CAD build for the part. Positions are in the model's coordinates, mm. A direction names the side the tool comes from. Coordinates: 2 decimals unless noted, no trailing zeros. Loops run counter-clockwise (first coordinate to the right, second up) from the corner with the lowest first, then second, coordinate; pieces in that order, holes last. Notation, with made-up numbers: (-33, 6.5) -> (-16, 6.5) arc R28 cw to (-16, 39.5) -> close; hole circle Ø5 at (78.25, 62.25). An arc over 180 degrees is marked (long way). Write each question's results on one line, items separated by ' | '.
from build123d import *

# Parameters (mm, degrees)
F0_W     = 74.25791291
F0_H     = 4.7
F0_W_2   = 3.271043545
F0_W_3   = 1.428956455
F0_H_2   = 8.3906837511
F0_H_3   = 13.5
F0_H_4   = 7.9193162489
F1_DEPTH = 27.2
F2_W     = 39.9343147874
F2_H     = 22.3026155613
F3_DEPTH = 155


with BuildPart() as f1:
    # F0 (on Top) → F1 (new body)
    with BuildSketch(Plane.XY):
        Polygon((-41.828956455, 87.5000014901), (-41.828956455, 74.9143162489), (-40.4, 74.9143162489), (-40.4, 83.305), (-37.128956455, 83.305), (-37.128956455, 87.5000014901), align=None)
        with Locations((0, 72.5643162489)):
            Rectangle(F0_W, F0_H)
        with Locations((-38.7644782275, 72.5643162489)):
            Rectangle(F0_W_2, F0_H)
        with Locations((-41.1144782275, 72.5643162489)):
            Rectangle(F0_W_3, F0_H)
        with Locations((38.7644782275, 79.1096581244)):
            Rectangle(F0_W_2, F0_H_2)
        Polygon((37.128956455, 87.5000014901), (37.128956455, 83.305), (40.4, 83.305), (40.4, 74.9143162489), (41.828956455, 74.9143162489), (41.828956455, 87.5000014901), align=None)
        with Locations((38.7644782275, 72.5643162489)):
            Rectangle(F0_W_2, F0_H)
        with Locations((41.1144782275, 72.5643162489)):
            Rectangle(F0_W_3, F0_H)
        with Locations((-41.1144782275, 63.4643162489)):
            Rectangle(F0_W_3, F0_H_3)
        with Locations((-38.7644782275, 63.4643162489)):
            Rectangle(F0_W_2, F0_H_3)
        with Locations((38.7644782275, 63.4643162489)):
            Rectangle(F0_W_2, F0_H_3)
        with Locations((41.1144782275, 63.4643162489)):
            Rectangle(F0_W_3, F0_H_3)
        with Locations((41.1144782275, 54.3643162489)):
            Rectangle(F0_W_3, F0_H)
        with Locations((38.7644782275, 54.3643162489)):
            Rectangle(F0_W_2, F0_H)
        with Locations((0, 54.3643162489)):
            Rectangle(F0_W, F0_H)
        with Locations((-41.1144782275, 54.3643162489)):
            Rectangle(F0_W_3, F0_H)
        with Locations((-38.7644782275, 54.3643162489)):
            Rectangle(F0_W_2, F0_H)
        with Locations((-41.1144782275, 45.2643162489)):
            Rectangle(F0_W_3, F0_H_3)
        with Locations((-38.7644782275, 45.2643162489)):
            Rectangle(F0_W_2, F0_H_3)
        with Locations((38.7644782275, 45.2643162489)):
            Rectangle(F0_W_2, F0_H_3)
        with Locations((41.1144782275, 45.2643162489)):
            Rectangle(F0_W_3, F0_H_3)
        with Locations((-41.1144782275, 36.1643162489)):
            Rectangle(F0_W_3, F0_H)
        with Locations((-38.7644782275, 36.1643162489)):
            Rectangle(F0_W_2, F0_H)
        with Locations((0, 36.1643162489)):
            Rectangle(F0_W, F0_H)
        with Locations((38.7644782275, 36.1643162489)):
            Rectangle(F0_W_2, F0_H)
        with Locations((41.1144782275, 36.1643162489)):
            Rectangle(F0_W_3, F0_H)
        with Locations((-41.1144782275, 27.0643162489)):
            Rectangle(F0_W_3, F0_H_3)
        with Locations((-38.7644782275, 27.0643162489)):
            Rectangle(F0_W_2, F0_H_3)
        with Locations((38.7644782275, 27.0643162489)):
            Rectangle(F0_W_2, F0_H_3)
        with Locations((41.1144782275, 27.0643162489)):
            Rectangle(F0_W_3, F0_H_3)
        with Locations((-41.1144782275, 17.9643162489)):
            Rectangle(F0_W_3, F0_H)
        with Locations((-38.7644782275, 17.9643162489)):
            Rectangle(F0_W_2, F0_H)
        with Locations((0, 17.9643162489)):
            Rectangle(F0_W, F0_H)
        with Locations((38.7644782275, 17.9643162489)):
            Rectangle(F0_W_2, F0_H)
        with Locations((41.1144782275, 17.9643162489)):
            Rectangle(F0_W_3, F0_H)
        with Locations((-41.1144782275, 8.8643162489)):
            Rectangle(F0_W_3, F0_H_3)
        with Locations((-38.7644782275, 8.8643162489)):
            Rectangle(F0_W_2, F0_H_3)
        with Locations((-41.1144782275, -0.2356837511)):
            Rectangle(F0_W_3, F0_H)
        with Locations((-38.7644782275, -0.2356837511)):
            Rectangle(F0_W_2, F0_H)
        with Locations((0, -0.2356837511)):
            Rectangle(F0_W, F0_H)
        with Locations((38.7644782275, 8.8643162489)):
            Rectangle(F0_W_2, F0_H_3)
        with Locations((41.1144782275, 8.8643162489)):
            Rectangle(F0_W_3, F0_H_3)
        with Locations((38.7644782275, -0.2356837511)):
            Rectangle(F0_W_2, F0_H)
        with Locations((41.1144782275, -0.2356837511)):
            Rectangle(F0_W_3, F0_H)
        with Locations((-41.1144782275, -9.3356837511)):
            Rectangle(F0_W_3, F0_H_3)
        with Locations((-38.7644782275, -9.3356837511)):
            Rectangle(F0_W_2, F0_H_3)
        with Locations((-41.1144782275, -18.4356837511)):
            Rectangle(F0_W_3, F0_H)
        with Locations((-38.7644782275, -18.4356837511)):
            Rectangle(F0_W_2, F0_H)
        with Locations((0, -18.4356837511)):
            Rectangle(F0_W, F0_H)
        with Locations((38.7644782275, -9.3356837511)):
            Rectangle(F0_W_2, F0_H_3)
        with Locations((41.1144782275, -9.3356837511)):
            Rectangle(F0_W_3, F0_H_3)
        with Locations((38.7644782275, -18.4356837511)):
            Rectangle(F0_W_2, F0_H)
        with Locations((41.1144782275, -18.4356837511)):
            Rectangle(F0_W_3, F0_H)
        with Locations((-41.1144782275, -27.5356837511)):
            Rectangle(F0_W_3, F0_H_3)
        with Locations((-38.7644782275, -27.5356837511)):
            Rectangle(F0_W_2, F0_H_3)
        with Locations((38.7644782275, -27.5356837511)):
            Rectangle(F0_W_2, F0_H_3)
        with Locations((41.1144782275, -27.5356837511)):
            Rectangle(F0_W_3, F0_H_3)
        with Locations((-41.1144782275, -36.6356837511)):
            Rectangle(F0_W_3, F0_H)
        with Locations((-38.7644782275, -36.6356837511)):
            Rectangle(F0_W_2, F0_H)
        with Locations((0, -36.6356837511)):
            Rectangle(F0_W, F0_H)
        with Locations((38.7644782275, -36.6356837511)):
            Rectangle(F0_W_2, F0_H)
        with Locations((41.1144782275, -36.6356837511)):
            Rectangle(F0_W_3, F0_H)
        with Locations((-41.1144782275, -45.7356837511)):
            Rectangle(F0_W_3, F0_H_3)
        with Locations((-38.7644782275, -45.7356837511)):
            Rectangle(F0_W_2, F0_H_3)
        with Locations((-41.1144782275, -54.8356837511)):
            Rectangle(F0_W_3, F0_H)
        with Locations((-38.7644782275, -54.8356837511)):
            Rectangle(F0_W_2, F0_H)
        with Locations((0, -54.8356837511)):
            Rectangle(F0_W, F0_H)
        with Locations((38.7644782275, -54.8356837511)):
            Rectangle(F0_W_2, F0_H)
        with Locations((41.1144782275, -54.8356837511)):
            Rectangle(F0_W_3, F0_H)
        with Locations((38.7644782275, -45.7356837511)):
            Rectangle(F0_W_2, F0_H_3)
        with Locations((41.1144782275, -45.7356837511)):
            Rectangle(F0_W_3, F0_H_3)
        with Locations((-41.1144782275, -63.9356837511)):
            Rectangle(F0_W_3, F0_H_3)
        with Locations((-38.7644782275, -63.9356837511)):
            Rectangle(F0_W_2, F0_H_3)
        with Locations((38.7644782275, -63.9356837511)):
            Rectangle(F0_W_2, F0_H_3)
        with Locations((41.1144782275, -63.9356837511)):
            Rectangle(F0_W_3, F0_H_3)
        with Locations((-41.1144782275, -73.0356837511)):
            Rectangle(F0_W_3, F0_H)
        with Locations((-38.7644782275, -73.0356837511)):
            Rectangle(F0_W_2, F0_H)
        with Locations((0, -73.0356837511)):
            Rectangle(F0_W, F0_H)
        with Locations((38.7644782275, -73.0356837511)):
            Rectangle(F0_W_2, F0_H)
        with Locations((41.1144782275, -73.0356837511)):
            Rectangle(F0_W_3, F0_H)
        Polygon((-41.828956455, -87.4999985099), (-37.128956455, -87.4999985099), (-37.128956455, -83.305), (-40.4, -83.305), (-40.4, -75.3856837511), (-41.828956455, -75.3856837511), align=None)
        with Locations((-38.7644782275, -79.3453418756)):
            Rectangle(F0_W_2, F0_H_4)
        with Locations((38.7644782275, -79.3453418756)):
            Rectangle(F0_W_2, F0_H_4)
        Polygon((40.4, -83.305), (37.128956455, -83.305), (37.128956455, -87.4999985099), (41.828956455, -87.4999985099), (41.828956455, -75.3856837511), (40.4, -75.3856837511), align=None)
        with Locations((-38.7644782275, 79.1096581244)):
            Rectangle(F0_W_2, F0_H_2)
    extrude(amount=F1_DEPTH)

    # F2 (on face) → F3 (cut)
    with BuildSketch(Plane.XZ.offset(75.3856837511)):
        with Locations((19.9671573937, 13.6)):
            Rectangle(F2_W, F2_H)
        with Locations((-19.9671573937, 13.6)):
            Rectangle(F2_W, F2_H)
    extrude(amount=-F3_DEPTH, mode=Mode.SUBTRACT)


solid = f1.part
1) Slice it at B-B (y = 6). Write the cut outline in (x, z).
Outcome:
outline: (-41.83, 0) -> (-37.13, 0) -> (-37.13, 2.45) -> (-39.93, 2.45) -> (-39.93, 24.75) -> (-37.13, 24.75) -> (-37.13, 27.2) -> (-41.83, 27.2) -> close; (37.13, 0) -> (41.83, 0) -> (41.83, 27.2) -> (37.13, 27.2) -> (37.13, 24.75) -> (39.93, 24.75) -> (39.93, 2.45) -> (37.13, 2.45) -> close
2) Slice it at C-C (x = -7). Count the separate pieces of the cut face and the enclosed holes in it, then the cut area to 3 significant figures.
Outcome:
separate pieces: 18 | enclosed holes: 0 | area: 207 mm^2
3) Pin check, flat tips, straight feed: pin 1 (0.7 mm diameter, centred on x = 10, z = 1, fed in from +Y); pin 2 (0.7 mm diameter, centred on x = 13, z = 26, fed in from -Y). Stop position of each tip, or through.
Outcome:
pin 1: stops at y = 74.91 | pin 2: stops at y = -75.39
4) Slice it at A-A (z = 9.75). Write the cut outline in (x, y), then the cut area to 3 significant figures.
Outcome:
outline: (-41.83, -87.5) -> (-37.13, -87.5) -> (-37.13, -75.39) -> (-39.93, -75.39) -> (-39.93, 79.61) -> (-37.13, 79.61) -> (-37.13, 87.5) -> (-41.83, 87.5) -> close; (37.13, -87.5) -> (41.83, -87.5) -> (41.83, 87.5) -> (37.13, 87.5) -> (37.13, 79.61) -> (39.93, 79.61) -> (39.93, -75.39) -> (37.13, -75.39) -> close | area: 775 mm^2
5) Two-plate mould, pull along Y, no slides. Class faces 4 (the flat face through (-40, -87.5, 13)), 5 (the flat face through (39.934, 1, 13)), 6 (the flat face through (37.129, 83, 13)): pulls with the +Y half, pulls with the -Y half, needs draft (parallel to the pull), parting line crosses it, or undercut.
Outcome:
face 4: pulls with the -Y half | face 5: undercut | face 6: needs draft
6) Which spindle directions (+Z, -Z, +X, -X, +Y, -Y) get a long thin tool onto all of the face, cutting with end or side? Do faces 1 (the flat face through (37.129, -81, 13)), 2 (the flat face through (-37.129, 83, 13)), 3 (the flat face through (-39.934, 1, 13)). Say none if no direction does.
Outcome:
face 1: +Z, -Z, -Y | face 2: +Z, -Z, +Y | face 3: none
7) Drill centre lines: L1, parallel to X at y = 8, z = 1.75; L2, parallel to X at y = -47, z = 20.25; L3, parallel to Z at x = -6, y = 2. Where is each one in solid material? Low to high. Write a range as from..to.
Outcome:
L1: x = -41.83..-37.13, 37.13..41.83 | L2: x = -41.83..-39.93, 39.93..41.83 | L3: z = 0..2.45, 24.75..27.2
